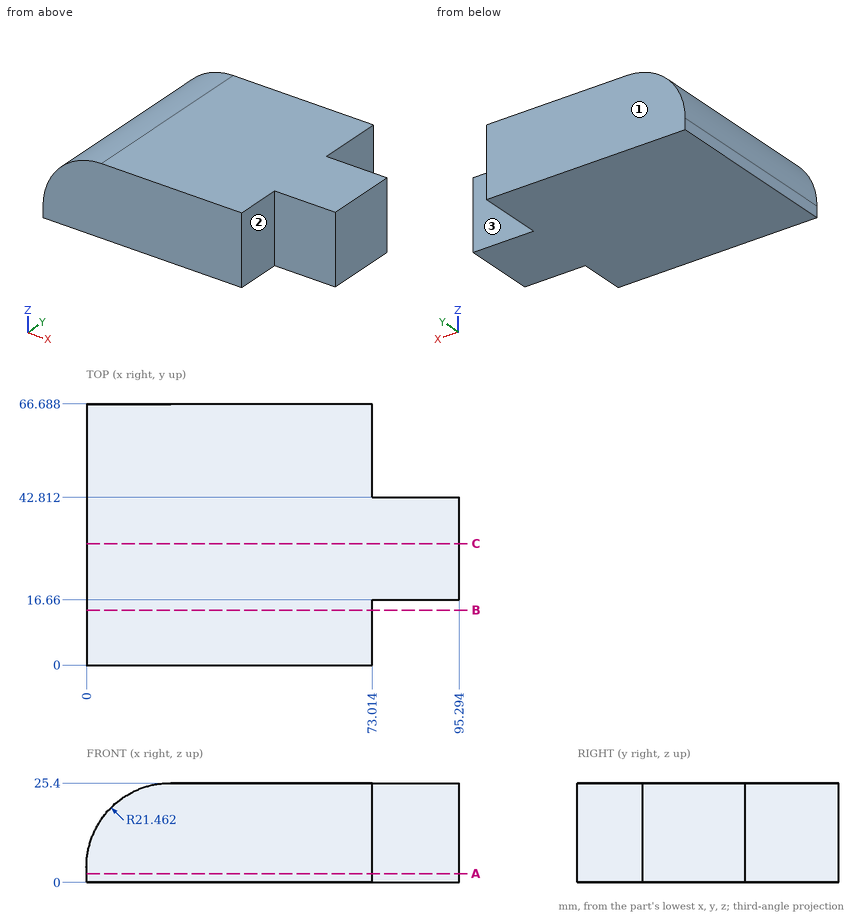
Source: three-view drawing plus pictorial views. Frame: mm from the lowest corner of the part. A direction names the side the tool comes from. Coordinates: 2 decimals unless noted, no trailing zeros. Order: outer loops, then holes, each group sorted by start corner. A loop starts at its lowest first (then second) coordinate and runs counter-clockwise, first axis right, second up. Notation, with made-up numbers: M 57.25,-16.5 L 100.25,-16.5 A14 ccw 100.25,-2.5 Z; hole C 10,9 d3. An arc over 180 degrees is marked long. Answer in a Markdown table with one row per item.
(1) Section query A-A, the plane z = 2.25. Output: boundary loops of the cut face in (x, y) (1 decimal).
Numbers:
| item | result |
|---|---|
| outline | M 0,0 L 73,0 L 73,16.7 L 95.3,16.7 L 95.3,42.8 L 73,42.8 L 73,66.7 L 0,66.7 Z |
(2) Section query C-C, the plane y = 31. Output: boundary loops of the cut face in (x, z) (1 decimal), plus the area to 3 significant figures.
Numbers:
| item | result |
|---|---|
| outline | M 0,0 L 95.3,0 L 95.3,25.4 L 21.5,25.4 A21.5 ccw 0,3.9 Z |
| area | 2,320 mm^2 |
(3) Material intervals for line 1 (X direction, y = 57, z = 3.75); line 2 (Y direction, x = 87.5, z = 18.5); line 3 (X direction, y = 47, z = 16) (1 decimal), sorted ascending. Write a range as [from, to].
Numbers:
| item | result |
|---|---|
| line 1 | x = [0, 73.01] |
| line 2 | y = [16.66, 42.81] |
| line 3 | x = [3.7, 73] |
(4) Section query B-B, the plane y = 14. Output: boundary loops of the cut face in (x, z) (1 decimal).
Numbers:
| item | result |
|---|---|
| outline | M 0,0 L 73,0 L 73,25.4 L 21.5,25.4 A21.5 ccw 0,3.9 Z |
(5) Contact query for flat-ended pins moving along their axis: pin 1 Ø8 at (y, z) = (42, 19.5) entering from -X; pin 2 Ø8 at (y, z) = (32.5, 4.5) entering from -X; pin 3 Ø5 at (y, z) = (37, 9) entering from -X; pin 4 Ø6.5 at (x, z) = (84.5, 14) entering from -Y. Output: stop coordinate, or through.
Numbers:
| item | result |
|---|---|
| pin 1 | stops at x = 3.38 |
| pin 2 | stops at x = 0 |
| pin 3 | stops at x = 0.15 |
| pin 4 | stops at y = 16.66 |
(6) Access query for the marked faces 1, 2 and 3. Directions: +Z, -Z, +X, -X, +Y, -Y. A direction counts if a zero-diameter tool reaches every point of the face in a straight line with its end or side. Return the directions, or none.
Numbers:
| item | result |
|---|---|
| face 1 | +Z, -Z, +X, -X, +Y |
| face 2 | +Z, -Z, +X, -Y |
| face 3 | +Z, -Z, +X, +Y |
